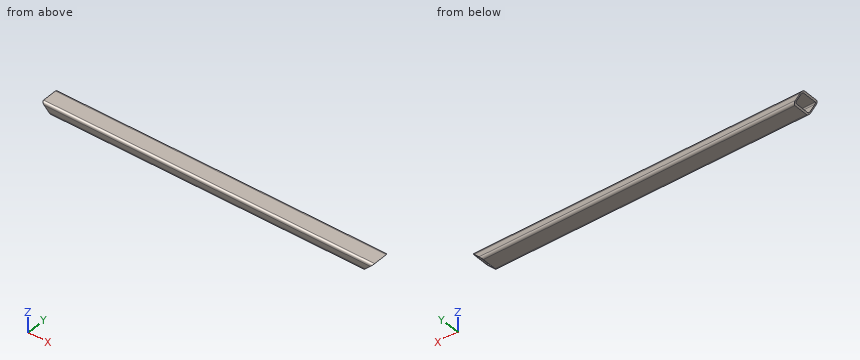
```python
from build123d import *

# Parameters (mm, degrees)
F1_DEPTH      = 215.9
F3_DEPTH      = 12.701
F3_DEPTH_BACK = 12.701


with BuildPart() as f1:
    # F0 (on Right) → F1 (new body, symmetric)
    with BuildSketch(Plane.YZ):
        with BuildLine():
            Line((-12.7, 3.175), (-12.7, -3.175))
            ThreePointArc((-12.7, -3.175), (-11.7700640303, -5.4200640303), (-9.525, -6.35))
            Line((-9.525, -6.35), (9.525, -6.35))
            ThreePointArc((9.525, -6.35), (11.7700640303, -5.4200640303), (12.7, -3.175))
            Line((12.7, -3.175), (12.7, 3.175))
            ThreePointArc((12.7, 3.175), (11.7700640303, 5.4200640303), (9.525, 6.35))
            Line((9.525, 6.35), (-9.525, 6.35))
            ThreePointArc((-9.525, 6.35), (-11.7700640303, 5.4200640303), (-12.7, 3.175))
        make_face()
        with BuildLine():
            ThreePointArc((-11.049, 3.175), (-10.6026307345, 4.2526307345), (-9.525, 4.699))
            Line((-9.525, 4.699), (9.525, 4.699))
            ThreePointArc((9.525, 4.699), (10.6026307345, 4.2526307345), (11.049, 3.175))
            Line((11.049, 3.175), (11.049, -3.175))
            ThreePointArc((11.049, -3.175), (10.6026307345, -4.2526307345), (9.525, -4.699))
            Line((9.525, -4.699), (-9.525, -4.699))
            ThreePointArc((-9.525, -4.699), (-10.6026307345, -4.2526307345), (-11.049, -3.175))
            Line((-11.049, -3.175), (-11.049, 3.175))
        make_face(mode=Mode.SUBTRACT)
    extrude(amount=F1_DEPTH, both=True)

    # F2 (on Front) → F3 (cut, two sides)
    with BuildSketch(Plane.XZ) as f3_sk:
        Polygon((-215.9, 6.35), (-215.9, -6.35), (-203.2, -6.35), align=None)
        Polygon((203.2, -6.35), (215.9, -6.35), (215.9, 6.35), align=None)
    extrude(amount=-F3_DEPTH, mode=Mode.SUBTRACT)
    extrude(f3_sk.sketch, amount=F3_DEPTH_BACK, mode=Mode.SUBTRACT)


solid = f1.part
```
Input: part model. Units: mm. Frame: model coordinates. Coordinates: 2 decimals unless noted, no trailing zeros. Loops run counter-clockwise (first coordinate to the right, second up) from the corner with the lowest first, then second, coordinate; pieces in that order, holes last. Notation, with made-up numbers: M -21,89 L -7,89 A20 cw -7,97 Z; hole C 57,50 d2. An arc over 180 degrees is marked long. One line per item, written item: value.
(1) Line query: line 1 along Z through (x, y) = (107, -3.75); line 2 along Z through (x, y) = (136.5, -10); line 3 along Y through (x, z) = (146, 2.5). Output: solid intervals per line, ascending. Write a range as from..to.
Filled in:
line 1: -6.35..-4.7, 4.7..6.35
line 2: -6.31..-4.62, 4.62..6.31
line 3: -12.7..-11.05, 11.05..12.7
(2) Section C-C (x = 147). Output: boundary loops of the cut face in (y, z) (3 decimals).
Filled in:
outline: M -12.7,-3.175 A3.175 ccw -9.525,-6.35 L 9.525,-6.35 A3.175 ccw 12.7,-3.175 L 12.7,3.175 A3.175 ccw 9.525,6.35 L -9.525,6.35 A3.175 ccw -12.7,3.175 Z; hole M -11.049,-3.175 A1.524 ccw -9.525,-4.699 L 9.525,-4.699 A1.524 ccw 11.049,-3.175 L 11.049,3.175 A1.524 ccw 9.525,4.699 L -9.525,4.699 A1.524 ccw -11.049,3.175 Z
(3) Section B-B (z = 0.25). Output: boundary loops of the cut face in (x, y).
Filled in:
outline: M -209.8,-12.7 L 209.8,-12.7 L 209.8,-11.05 L -209.8,-11.05 Z; M -209.8,11.05 L 209.8,11.05 L 209.8,12.7 L -209.8,12.7 Z
(4) Section A-A (y = -6). Output: boundary loops of the cut face in (x, z).
Filled in:
outline: M -215.9,6.35 L -214.25,4.7 L 214.25,4.7 L 215.9,6.35 Z; M -204.85,-4.7 L -203.2,-6.35 L 203.2,-6.35 L 204.85,-4.7 Z
(5) Pin query (flat end, axial travel): pin 1 (3 mm diameter, centred on y = -1, z = -4.5, fed in from -X). Return the tip coordinate at first contact, or that it passes through.
Filled in:
pin 1: x = -204.85
